Geometry check sheet. Reference: the model listing, model coordinates, mm. Face numbers are marked on the shaded views. A direction names the side the tool comes from. Round coordinates to 2 decimals unless told otherwise and drop trailing zeros. Write each loop counter-clockwise with the first axis right and the second up, starting at its lowest first coordinate (ties: lowest second). Pieces come first, ordered by that corner, then holes. Notation, with made-up numbers: M -14,82 L 5,82 A17 ccw 5,96 Z; hole C 57,-37.75 d7. An arc over 180 degrees is marked long. Use a Markdown table: item, result.
```python
from build123d import *

# Parameters (mm, degrees)
PAD_DEPTH    = 3.5
SKETCH001_W  = 15
SKETCH001_H  = 6.5
SKETCH001_R  = 1.55
PAD001_DEPTH = 5
SKETCH002_W  = 5.6
SKETCH002_H  = 5.6
POCKET_DEPTH = 2
SKETCH003_R  = 1.6
PAD002_DEPTH = 7.5
FILLET_R     = 1.5
FILLET001_R  = 1.1
FILLET002_R  = 1


with BuildPart() as part:
    # Sketch → Pad (new body)
    with BuildSketch(Plane.XZ):
        with BuildLine():
            Line((14, -8), (14, -15))
            Line((14, -15), (19, -15))
            Line((19, -15), (19, 0))
            Line((6.1, 0), (19, 0))
            ThreePointArc((3.1, 3), (3.97868, 0.87868), (6.1, 0))
            Line((3.1, 5), (3.1, 3))
            Line((-3.1, 5), (3.1, 5))
            Line((-3.1, -1.9), (-3.1, 5))
            ThreePointArc((-3.1, -1.9), (-2.192031, -4.092031), (0, -5))
            Line((11, -5), (0, -5))
            ThreePointArc((14, -8), (13.12132, -5.87868), (11, -5))
        make_face()
    extrude(amount=PAD_DEPTH)

    # Sketch001 (on Face4 of Pad) → Pad001 (join)
    with BuildSketch(Plane(origin=(19, 0, 0), x_dir=(0, 0, 1), z_dir=(1, 0, 0))):
        with Locations((-7.5, -3.25)):
            Rectangle(SKETCH001_W, SKETCH001_H)
        with Locations((-4, -3.7)):
            Circle(SKETCH001_R, mode=Mode.SUBTRACT)
        with Locations((-11, -3.7)):
            Circle(SKETCH001_R, mode=Mode.SUBTRACT)
    extrude(amount=-PAD001_DEPTH)

    # Sketch002 (on Face10 of Pad001) → Pocket (cut)
    with BuildSketch(Plane(origin=(14, 0, 0), x_dir=(0, 0, -1), z_dir=(-1, 0, 0))):
        with Locations((4, -3.7)):
            Rectangle(SKETCH002_W, SKETCH002_H)
        with Locations((11, -3.7)):
            Rectangle(SKETCH002_W, SKETCH002_H)
    extrude(amount=-POCKET_DEPTH, mode=Mode.SUBTRACT)

    # Sketch003 (on Face4 of Pocket) → Pad002 (join)
    with BuildSketch(Plane(origin=(0, 0, 0), x_dir=(1, 0, 0), z_dir=(0, 1, 0))):
        with Locations((0, 2.25)):
            Circle(SKETCH003_R)
        with Locations((0, -2.25)):
            Circle(SKETCH003_R)
    extrude(amount=PAD002_DEPTH)

    # Fillet
    fillet_edges = [part.edges().sort_by_distance(p)[0] for p in [
        (-3.1, -1.75, 5),
        (3.1, -1.75, 5),
    ]]
    fillet(fillet_edges, radius=FILLET_R)

    # Fillet001
    fillet001_edges = [part.edges().sort_by_distance(p)[0] for p in [
        (10.05, 0, 0),
        (3.97868, 0, 0.87868),
        (3.1, 0, 3.25),
        (2.66066, 0, 4.56066),
        (0, 0, 5),
        (-2.66066, 0, 4.56066),
        (-3.1, 0, 0.8),
        (-2.192031, 0, -4.092031),
        (5.5, 0, -5),
        (13.12132, 0, -5.87868),
    ]]
    fillet(fillet001_edges, radius=FILLET001_R)

    # Fillet002
    fillet002_edges = [part.edges().sort_by_distance(p)[0] for p in [
        (-1.6, 7.5, 2.25),
        (-1.6, 7.5, -2.25),
    ]]
    fillet(fillet002_edges, radius=FILLET002_R)


solid = part.part
```
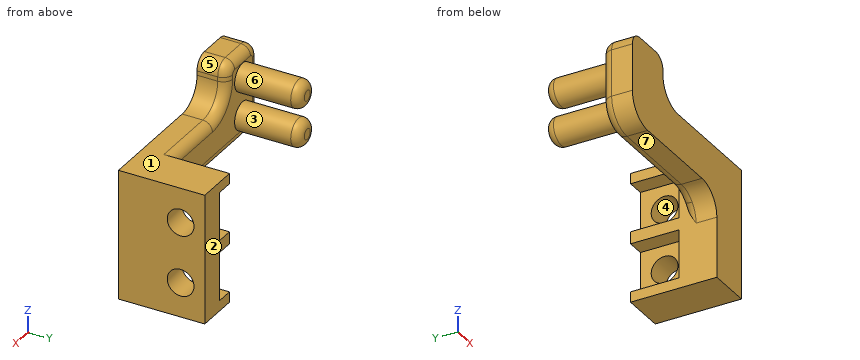
Item 1: Mould release check, pull along Z, two halves, no side actions. Record for the marked faces 5, 6 and 7: +Z half, -Z half, draft (parallel to the pull), parting line (faces both ways), or undercut.
Outcome:
| item | result |
|---|---|
| face 5 | +Z half |
| face 6 | undercut |
| face 7 | -Z half |
Item 2: Material ranges on line 1 along Z through (x, y) = (18.3, 3.7); line 2 along Y through (x, z) = (17.5, -11); line 3 along Z through (x, y) = (0.75, 1.75), recorded low to high. Write a range as from..to.
Outcome:
| item | result |
|---|---|
| line 1 | z = -15..-12.55, -9.45..-5.55, -2.45..0 |
| line 2 | y = -3.5..2.15, 5.25..6.5 |
| line 3 | z = -3.66..-0.84, 0.84..3.66 |
Item 3: Access from +Z, -Z, +X, -X, +Y, -Y to the whole of each face (thin tool, end or side, straight path). Record for the marked faces 1, 2, 3 and 4.
Outcome:
| item | result |
|---|---|
| face 1 | +Z, +X, +Y, -Y |
| face 2 | +Z, -Z, +X, +Y |
| face 3 | +Y |
| face 4 | +X |
Item 4: Go/stop test with flat-tipped pins: pin 1 (4 mm diameter, centred on x = 4, z = 2, fed in from +Y); pin 2 (2.5 mm diameter, centred on x = 17, z = -10.5, fed in from +Y); pin 3 (0.7 mm diameter, centred on x = 3.5, y = -2, fed in from -Z); pin 4 (3.5 mm diameter, centred on y = 3.7, z = -11, fed in from +X). Record where each tip stops, or that it passes through.
Outcome:
| item | result |
|---|---|
| pin 1 | stops at y = 0 |
| pin 2 | stops at y = 6.5 |
| pin 3 | stops at z = -5 |
| pin 4 | stops at x = 19 |
Item 5: Cross-section at A-A, the plane z = -11. Record the cut outline in (x, y).
Outcome:
| item | result |
|---|---|
| outline | M 14,-3.5 L 19,-3.5 L 19,2.15 L 16,2.15 L 16,0.9 L 14,0.9 Z; M 16,5.25 L 19,5.25 L 19,6.5 L 16,6.5 Z |
Item 6: Cross-section at B-B, the plane y = -1.5. Record the cut outline in (x, z), and give its area (3 significant figures).
Outcome:
| item | result |
|---|---|
| outline | M -3.1,-1.9 A3.1 ccw 0,-5 L 11,-5 A3 cw 14,-8 L 14,-15 L 19,-15 L 19,0 L 6.1,0 A3 cw 3.1,3 L 3.1,3.5 A1.5 ccw 1.6,5 L -1.6,5 A1.5 ccw -3.1,3.5 Z |
| area | 192 mm2 |
